The drawing under review shows one solid part. Ordinate dimensions are in mm from its lowest x, y, z. A direction names the side the tool comes from. Coordinates: 2 decimals unless noted, no trailing zeros. Loops run counter-clockwise (first coordinate to the right, second up) from the corner with the lowest first, then second, coordinate; pieces in that order, holes last. Notation, with made-up numbers: (-25.5, -18.75) - (23.5, -18.75) arc R10 cw to (23.5, -12.75) - close; hole circle Ø9 at (56.5, 77). An arc over 180 degrees is marked (long way). Use one line per item in the form item = value. Start each with the question number.
1. For pin 1 Ø18 at (x, z) = (38.1, 19.05) entering from +Y; pin 2 Ø12 at (y, z) = (15.5, 23) entering from -X, all flat-tipped, find the tip position at first contact; note any pin that passes through.
2. Add section A-A on y = 9.75. Give the boundary of the cut face in (x, z).
3. To check wall thickness, follow probe 1 along Y at (x, z) = (36.5, 2); probe 2 along Z at (x, y) = (31.5, 11); probe 3 along X at (y, z) = (24.35, 19.05). State the ranges of each line that lie inside material, in increasing order.
4. Machinability: for the marked faces 1 and 2, which of the approach directions +Z, -Z, +X, -X, +Y, -Y give a long, thin tool a straight path to every point of the face, cutting with its end or side? Answer none if there is none.
5. Draft analysis for pull direction Z (two halves, no side actions). For the marked faces 3, 4, 5 and 6, state which applies: +Z half, -Z half, draft (parallel to the pull), parting line (faces both ways), or undercut.
6. Add section C-C on x = 20. Give the boundary of the cut face in (y, z).
7. Add section D-D on z = 34. Give the boundary of the cut face in (x, y).
8. Add section B-B on z = 19.05. Give the boundary of the cut face in (x, y), and give its area (3 significant figures).
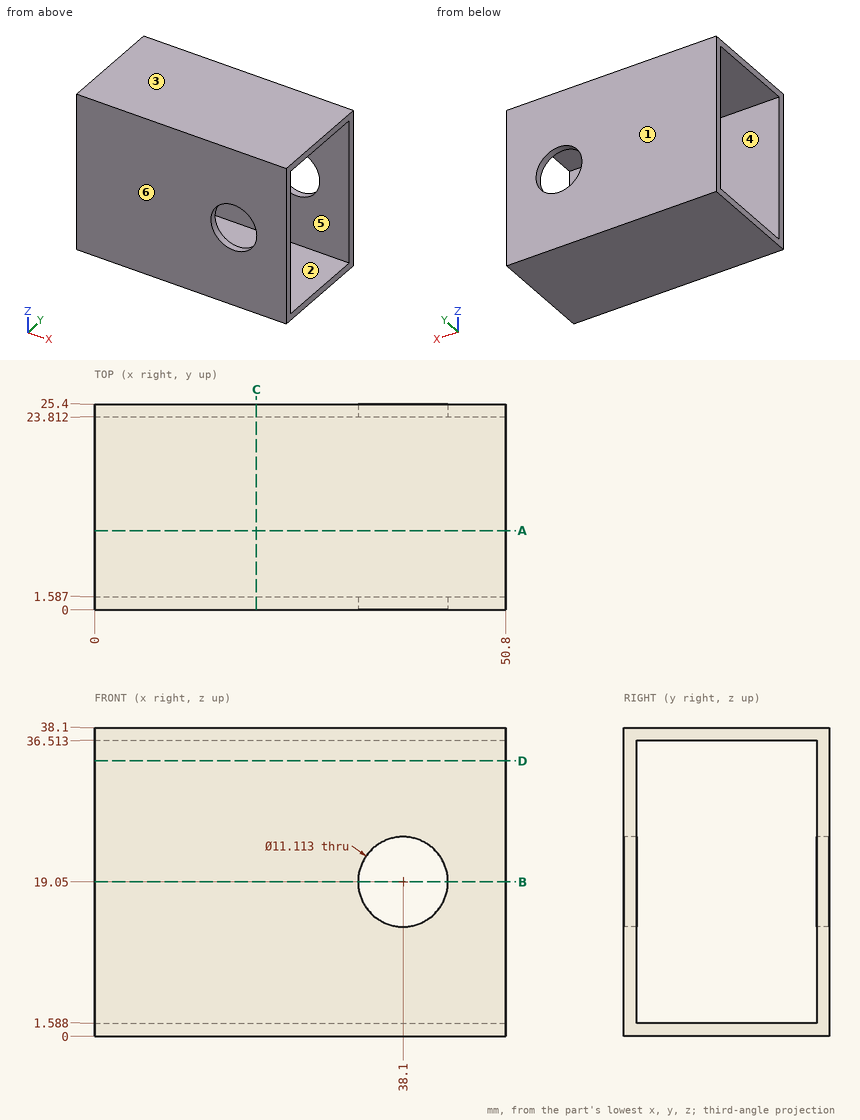
Conclusion:
q1.pin_1 = 25.4
q1.pin_2 = through
q2.outline = (0, 0) - (50.8, 0) - (50.8, 1.59) - (0, 1.59) - close; (0, 36.51) - (50.8, 36.51) - (50.8, 38.1) - (0, 38.1) - close
q3.probe_1 = 0 to 1.59, 23.81 to 25.4
q3.probe_2 = 0 to 1.59, 36.51 to 38.1
q3.probe_3 = 0 to 32.54, 43.66 to 50.8
q4.face_1 = +Z, -Z, +X, -X, +Y
q4.face_2 = +X, -X
q5.face_3 = +Z half
q5.face_4 = undercut
q5.face_5 = undercut
q5.face_6 = draft
q6.outline = (0, 0) - (25.4, 0) - (25.4, 38.1) - (0, 38.1) - close; hole (1.59, 1.59) - (23.81, 1.59) - (23.81, 36.51) - (1.59, 36.51) - close
q7.outline = (0, 0) - (50.8, 0) - (50.8, 1.59) - (0, 1.59) - close; (0, 23.81) - (50.8, 23.81) - (50.8, 25.4) - (0, 25.4) - close
q8.outline = (0, 0) - (32.54, 0) - (32.54, 1.59) - (0, 1.59) - close; (0, 23.81) - (32.54, 23.81) - (32.54, 25.4) - (0, 25.4) - close; (43.66, 0) - (50.8, 0) - (50.8, 1.59) - (43.66, 1.59) - close; (43.66, 23.81) - (50.8, 23.81) - (50.8, 25.4) - (43.66, 25.4) - close
q8.area = 126 mm^2
